Read the model definition and answer for the solid it produces. Units are mm, in the model's axes. A direction names the side the tool comes from. Round coordinates to 2 decimals unless told otherwise and drop trailing zeros. Order: outer loops, then holes, each group sorted by start corner. A loop starts at its lowest first (then second) coordinate and runs counter-clockwise, first axis right, second up. Notation, with made-up numbers: (0.25, 57.25) -> (35.25, 57.25) arc R24 ccw to (35.25, 71.25) -> close; hole circle Ø2 at (6, 22.5). An arc over 180 degrees is marked (long way). Use a Markdown table: item, result. Add a question column.
1. Given pin 1 (1.5 mm diameter, centred on x = 3, z = -42, fed in from +Y); pin 2 (3.5 mm diameter, centred on x = 3.5, z = -2.5, fed in from -Y); pin 3 (12 mm diameter, centred on y = 6.5, z = -19.5, fed in from +X), each flat-ended and moving along its own axis, determine where each tip first touches the part or whether it passes through.
2. Consider L1, parallel to X at y = 21, z = -106; L2, parallel to X at y = 26.5, z = -2.5; L3, parallel to X at y = 28, z = -41.5. Determine where each line is inside the solid, lowest interval first. Write a range as [from, to].
3. The mould has two halves that part along X. Classify faces 1 (the face through (2.6, 1.4, -1.6)), 2 (the face through (2.6, 1.4, -40.6)), 3 (the face through (5.287, 1.47, -4.248)), 4 (the face through (-2, 29, -72)): +X half, -X half, draft (parallel to the pull), parting line (faces both ways), or undercut.
4. Section B-B, the plane z = -71 is taken. Give the vertices of the cut face in (x, y).
5. Section A-A, the plane y = 11.5 is taken. Give the vertices of the cut face in (x, z), then the cut area to 3 significant figures.
6. For faces 5 (the face through (5.287, 1.47, -39.752)), 6 (the face through (2.6, 27.6, -1.6)), 7 (the face through (2, 1, -44)), 8 (the face through (2, 26.1, -2)), 9 (the face through (4.852, 0.69, -3.974)), determine the directions among +Z, -Z, +X, -X, +Y, -Y from which every point of the face is accessible in a straight line to the end or side of a thin tool.
```python
from build123d import *

# Parameters (mm, degrees)
SKETCH1_W           = 5
SKETCH1_H           = 150
BOSS_EXTRUDE1_DEPTH = 29
SKETCH2_W           = 5
SKETCH2_H           = 2.9
BOSS_EXTRUDE2_DEPTH = 6
SKETCH3_R           = 1.05
CUT_EXTRUDE1_DEPTH  = 153.895389074
SKETCH4_R           = 2
CUT_EXTRUDE2_DEPTH  = 1.4
FILLET1_R           = 4
FILLET2_R           = 2.5


with BuildPart() as part:
    # Sketch1 → Boss-Extrude1 (new body)
    with BuildSketch(Plane(origin=(0, 0, 0), x_dir=(1, 0, 0), z_dir=(0, 1, 0))):
        with Locations((-2.5, 75)):
            Rectangle(SKETCH1_W, SKETCH1_H)
    extrude(amount=BOSS_EXTRUDE1_DEPTH)

    # Sketch2 → Boss-Extrude2 (add)
    with BuildSketch(Plane(origin=(0, 0, 0), x_dir=(0, 0, -1), z_dir=(1, 0, 0))):
        with Locations((2.5, 27.55)):
            Rectangle(SKETCH2_W, SKETCH2_H)
        with Locations((41.5, 27.55)):
            Rectangle(SKETCH2_W, SKETCH2_H)
        with Locations((41.5, 1.45)):
            Rectangle(SKETCH2_W, SKETCH2_H)
        with Locations((2.5, 1.45)):
            Rectangle(SKETCH2_W, SKETCH2_H)
    extrude(amount=BOSS_EXTRUDE2_DEPTH)

    # Sketch3 → Cut-Extrude1 (cut, through all)
    with BuildSketch(Plane(origin=(0, 29, 0), x_dir=(1, 0, 0), z_dir=(0, 1, 0))):
        with Locations(Location((3.5, 41.5, 0), (0, 0, 270))):
            Circle(SKETCH3_R)
        with Locations(Location((3.5, 2.5, 0), (0, 0, 270))):
            Circle(SKETCH3_R)
    extrude(amount=-CUT_EXTRUDE1_DEPTH, mode=Mode.SUBTRACT)

    # Sketch4 → Cut-Extrude2 (cut)
    with BuildSketch(Plane(origin=(0, 29, 0), x_dir=(1, 0, 0), z_dir=(0, 1, 0))):
        with Locations(Location((3.5, 41.5, 0), (0, 0, 270))):
            Circle(SKETCH4_R)
        with Locations(Location((3.5, 2.5, 0), (0, 0, 270))):
            Circle(SKETCH4_R)
    cut_extrude2 = extrude(amount=-CUT_EXTRUDE2_DEPTH, mode=Mode.SUBTRACT)

    # Mirror2: Cut-Extrude2 across plane
    add(cut_extrude2.mirror(Plane.ZX.offset(14.5)), mode=Mode.SUBTRACT)

    # Fillet1
    fillet1_edges = [part.edges().sort_by_distance(p)[0] for p in [
        (-2.5, 0, -150),
        (-5, 14.5, 0),
        (-2.5, 29, -150),
    ]]
    fillet(fillet1_edges, radius=FILLET1_R)

    # Fillet2
    fillet2_edges = [part.edges().sort_by_distance(p)[0] for p in [
        (6, 1.45, -5),
        (6, 1.45, 0),
        (6, 1.45, -44),
        (6, 1.45, -39),
        (6, 27.55, -44),
        (6, 27.55, -39),
        (6, 27.55, -5),
        (6, 27.55, 0),
    ]]
    fillet(fillet2_edges, radius=FILLET2_R - 0.0001)  # a hair under: the kernel refuses the full size


solid = part.part
```
Verdict:
| question | item | result |
|---|---|---|
| 1 | pin 1 | stops at y = 27.6 |
| 1 | pin 2 | stops at y = 1.4 |
| 1 | pin 3 | stops at x = 0 |
| 2 | L1 | x = [-5, 0] |
| 2 | L2 | x = [-4.71, 2.45], [4.55, 6] |
| 2 | L3 | x = [-5, 1.5], [5.5, 6] |
| 3 | face 1 | undercut |
| 3 | face 2 | undercut |
| 3 | face 3 | +X half |
| 3 | face 4 | draft |
| 4 | outline | (-5, 0) -> (0, 0) -> (0, 29) -> (-5, 29) -> close |
| 5 | outline | (-5, -150) -> (0, -150) -> (0, 0) -> (-1, 0) arc R4 ccw to (-5, -4) -> close |
| 5 | area | 747 mm2 |
| 6 | face 5 | +X, +Y, -Y |
| 6 | face 6 | +Y |
| 6 | face 7 | -Z, +X, +Y, -Y |
| 6 | face 8 | +Z, -Z, +X |
| 6 | face 9 | -Y |
